```python
from build123d import *

# Parameters (mm, degrees)
F0_W     = 70
F0_H     = 115
F1_DEPTH = 6.5
F2_W     = 10.5
F2_H     = 24.5
F3_DEPTH = 6.5
F4_R     = 3


with BuildPart() as f1:
    # F0 (on Top) → F1 (new body)
    with BuildSketch(Plane.XY):
        with Locations((0.0314470381, -4.1025115179)):
            Rectangle(F0_W, F0_H)
    extrude(amount=F1_DEPTH)

    # F2 (on face) → F3 (cut, through all)
    with BuildSketch(Plane.XY.offset(6.5)):
        with Locations((0.6114470381, -4.1025115179)):
            Rectangle(F2_W, F2_H)
    extrude(amount=-F3_DEPTH, mode=Mode.SUBTRACT)

    # F4
    f4_edges = [f1.edges().sort_by_distance(p)[0] for p in [
        (35.031447, -4.102512, 6.5),
        (0.031447, -61.602512, 6.5),
        (0.031447, 53.397488, 6.5),
        (-34.968553, -4.102512, 6.5),
        (-4.638553, -4.102512, 6.5),
        (0.611447, -16.352512, 6.5),
        (5.861447, -4.102512, 6.5),
        (0.611447, 8.147488, 6.5),
    ]]
    fillet(f4_edges, radius=F4_R)


solid = f1.part
```
The model under review builds one solid part; all positions refer to its coordinate system, in mm. A direction names the side the tool comes from. Round coordinates to 2 decimals unless told otherwise and drop trailing zeros. Loops run counter-clockwise (first coordinate to the right, second up) from the corner with the lowest first, then second, coordinate; pieces in that order, holes last. Notation, with made-up numbers: (44, 79.25) - (91, 79.25) arc R33 ccw to (91, 108.25) - close; hole circle Ø10 at (-15, -21). An arc over 180 degrees is marked (long way). Write each question's results on one line, items separated by ' | '. Start each with the question number.
Q1. Take a section at D-D on x = -6. Give the boundary of the cut face in (y, z).
Q2. Take a section at C-C on z = 1.25. Give the boundary of the cut face in (x, y).
Q3. Take a section at B-B on x = 3. Give the boundary of the cut face in (y, z), plus the area to 3 significant figures.
Q4. Tool access review of faces 4 (the cylindrical face through (0.727, 9.454, 5.976)), 5 (the flat face through (1, -16.353, 2)), 6 (the flat face through (-34.969, -5, 2)): name each direction out of +Z, -Z, +X, -X, +Y, -Y from which nothing blocks a thin tool from reaching the whole face with its end or side.
Q5. Wall thickness on line 1 along X through (y, z) = (7, 1.5); line 2 along Y through (x, z) = (-2, 2); line 3 along X through (y, z) = (-16, 5): over which ranges is each line inside the solid? List them lowest first. Write a range as [from, to].
Q6. Take a section at A-A on y = -4.5. Give the boundary of the cut face in (x, z), plus the area to 3 significant figures.
Q7. Draft analysis for pull direction X (two halves, no side actions). For faces 1 (the cylindrical face through (-34.11, -3.3, 5.6)), 2 (the flat face through (-4.639, -4, 2)), 3 (the flat face through (0, 53.397, 2)), state which applies: pulls with the +X half, pulls with the -X half, needs draft (parallel to the pull), parting line crosses it, or undercut.
Data:
1) outline: (-61.6, 0) - (53.4, 0) - (53.4, 3.5) arc R3 ccw to (50.4, 6.5) - (11.15, 6.5) arc R3 ccw to (9.51, 6.01) - (-17.71, 6.01) arc R3 ccw to (-19.35, 6.5) - (-58.6, 6.5) arc R3 ccw to (-61.6, 3.5) - close
2) outline: (-34.97, -61.6) - (35.03, -61.6) - (35.03, 53.4) - (-34.97, 53.4) - close; hole (-4.64, -16.35) - (5.86, -16.35) - (5.86, 8.15) - (-4.64, 8.15) - close
3) outline: (-61.6, 0) - (-16.35, 0) - (-16.35, 3.5) arc R3 ccw to (-19.35, 6.5) - (-58.6, 6.5) arc R3 ccw to (-61.6, 3.5) - close; (8.15, 0) - (53.4, 0) - (53.4, 3.5) arc R3 ccw to (50.4, 6.5) - (11.15, 6.5) arc R3 ccw to (8.15, 3.5) - close | area: 581 mm²
4) face 4: +Z | face 5: +Z, -Z | face 6: +Z, -Z, -X, +Y, -Y
5) line 1: x = [-34.97, -4.64], [5.86, 35.03] | line 2: y = [-61.6, -16.35], [8.15, 53.4] | line 3: x = [-34.57, -5.04], [6.26, 34.63]
6) outline: (-34.97, 0) - (-4.64, 0) - (-4.64, 3.5) arc R3 ccw to (-7.64, 6.5) - (-31.97, 6.5) arc R3 ccw to (-34.97, 3.5) - close; (5.86, 0) - (35.03, 0) - (35.03, 3.5) arc R3 ccw to (32.03, 6.5) - (8.86, 6.5) arc R3 ccw to (5.86, 3.5) - close | area: 379 mm²
7) face 1: pulls with the -X half | face 2: undercut | face 3: needs draft
